Part model, mm, in its own coordinate system. A direction names the side the tool comes from. Round coordinates to 2 decimals unless told otherwise and drop trailing zeros. Order: outer loops, then holes, each group sorted by start corner. A loop starts at its lowest first (then second) coordinate and runs counter-clockwise, first axis right, second up. Notation, with made-up numbers: (-13, -31) - (-7, -31) arc R32 ccw to (-7, 1) - close; hole circle Ø7 at (15, 31). An arc over 180 degrees is marked (long way). Return JSON: item names as keys, results as strings. Group by question number.
Item 1: Probe probe 1 along X at (y, z) = (43.2, 0); probe 2 along Y at (x, z) = (-4.5, -9.5); probe 3 along Y at (x, z) = (-35.5, -7). List the from-to ranges inside material, lowest first.
Item 2: Two-plate mould, pull along Z, no slides. Class faces 4 (the face through (-76.22, 42.46, 1.15)), 5 (the face through (-19, 31, 0)), 6 (the face through (-48, 42, -18)), 7 (the face through (-3, 32, 21)): released by +Z, released by -Z, zero draft, split by the parting line, or undercut.
Item 3: Saw through at B-B on y = 35.5. List the corners of the cut face in (x, z), and give its area (3 significant figures).
Item 4: Saw through at A-A on x = -49. List the corners of the cut face in (y, z), and give its area (3 significant figures).
Item 5: Drop flat-ended pins along their axis: pin 1 (10 mm diameter, centred on y = 2.5, z = 9.5, fed in from -X); pin 2 (2 mm diameter, centred on y = 34.5, z = 20, fed in from -X); pin 3 (5 mm diameter, centred on x = -64.5, y = 41.5, fed in from -Z). Give the stop position or say it passes through.
Item 6: Saw through at D-D on y = 46. List the corners of the cut face in (x, z), and give its area (3 significant figures).
Item 7: Saw through at C-C on x = -70. List the corners of the cut face in (y, z), and give its area (3 significant figures).
Item 8: Tool access for faces 1 (the face through (-80, 42, 0)), 2 (the face through (-22.994, 30.524, -0.506)), 3 (the face through (-6, 32, 20)): list every direction of +Z, -Z, +X, -X, +Y, -Y with a clear straight run to the whole face (end or side of a thin tool).
```python
from build123d import *

# Parameters (mm, degrees)
BOSS_EXTRUDE1_DEPTH     = 62
BOSS_EXTRUDE2_START     = 3
BOSS_EXTRUDE2_DEPTH     = 3
SKETCH4_R               = 5
BOSS_EXTRUDE3_DEPTH     = 5
M6X1_0_TAPPED_HOLE1_D   = 5
CUT_EXTRUDE1_DEPTH      = 71.014284257
CUT_EXTRUDE1_DEPTH_BACK = 71.014284257
SKETCH8_W               = 3
SKETCH8_H               = 20
BOSS_EXTRUDE4_DEPTH     = 3
CUT_EXTRUDE2_REACH      = 81.919
SKETCH11_R              = 2.5
BOSS_EXTRUDE5_DEPTH     = 5
FILLET1_R               = 2


with BuildPart() as part:
    # Sketch1 → Boss-Extrude1 (new body)
    with BuildSketch(Plane(origin=(0, 0, 0), x_dir=(1, 0, 0), z_dir=(0, 1, 0))):
        with BuildLine():
            Line((0, 23), (0, 19))
            ThreePointArc((0, 19), (-19, 0), (0, -19))
            Line((0, -19), (0, -23))
            ThreePointArc((0, -23), (-23, 0), (0, 23))
        make_face()
    extrude(amount=BOSS_EXTRUDE1_DEPTH)

    # Sketch3 → Boss-Extrude2 (add)
    with BuildSketch(Plane.XZ.offset(BOSS_EXTRUDE2_START)):
        with BuildLine():
            Line((0, 23), (0, 3.75))
            ThreePointArc((0, 3.75), (-3.75, 0), (0, -3.75))
            Line((0, -3.75), (0, -23))
            ThreePointArc((0, -23), (-23, 0), (0, 23))
        make_face()
    extrude(amount=-BOSS_EXTRUDE2_DEPTH)

    # Sketch4 → Boss-Extrude3 (add)
    with BuildSketch(Plane.XZ.offset(3)):
        with Locations(Location((-10, 0, 0), (0, 0, 270))):
            Circle(SKETCH4_R)
    extrude(amount=BOSS_EXTRUDE3_DEPTH)

    # M6x1.0 Tapped Hole1 (through all)
    with Locations(Plane.XZ.offset(8)):
        with Locations((-10, 0)):
            Hole(M6X1_0_TAPPED_HOLE1_D / 2)

    # Sketch8 → Cut-Extrude1 (cut, two sides: drawn at the far end of the back side and taken through both)
    with BuildSketch(Plane.XY.offset(-CUT_EXTRUDE1_DEPTH_BACK)):
        with Locations((-4.5, 32)):
            Rectangle(SKETCH8_W, SKETCH8_H)
    extrude(amount=CUT_EXTRUDE1_DEPTH + CUT_EXTRUDE1_DEPTH_BACK, mode=Mode.SUBTRACT)

    # Sketch9 → Boss-Extrude4 (add)
    with BuildSketch(Plane(origin=(0, 62, 0), x_dir=(1, 0, 0), z_dir=(0, 1, 0))):
        with BuildLine():
            Line((0, -23), (0, 23))
            ThreePointArc((0, 23), (-23, 0), (0, -23))
        make_face()
    extrude(amount=BOSS_EXTRUDE4_DEPTH)

    # Sketch10 → Cut-Extrude2 (cut, up to next)
    with BuildSketch(Plane(origin=(0, 65, 0), x_dir=(1, 0, 0), z_dir=(0, 1, 0)), mode=Mode.PRIVATE) as cut_extrude2_sk1:
        with BuildLine():
            Line((0, -5), (-12, -5))
            ThreePointArc((-12, -5), (-17, 0), (-12, 5))
            Line((-12, 5), (0, 5))
            ThreePointArc((0, 5), (5, 0), (0, -5))
        make_face()
    cut_extrude2_tool1 = extrude(cut_extrude2_sk1.sketch, amount=-CUT_EXTRUDE2_REACH, mode=Mode.PRIVATE) & part.part
    add(cut_extrude2_tool1.solids().sort_by_distance((-6, 65, 0))[0], mode=Mode.SUBTRACT)

    # Sketch11 → Boss-Extrude5 (add)
    with BuildSketch(Plane(origin=(0, 40, 0), x_dir=(-1, 0, 0), z_dir=(0, 1, 0))):
        with BuildLine():
            Line((14.317821063, 18), (80, 18))
            Line((80, 18), (80, -18))
            Line((80, -18), (14.317821063, -18))
            ThreePointArc((14.317821063, -18), (23, 0), (14.317821063, 18))
        make_face()
        with Locations(Location((49, 0, 0), (0, 0, 90))):
            Circle(SKETCH11_R, mode=Mode.SUBTRACT)
        with Locations(Location((74, 0, 0), (0, 0, 90))):
            Circle(SKETCH11_R, mode=Mode.SUBTRACT)
    extrude(amount=BOSS_EXTRUDE5_DEPTH)

    # Fillet1
    fillet1_edges = [part.edges().sort_by_distance(p)[0] for p in [
        (-23, 40, 0),
        (-23, 45, 0),
    ]]
    fillet(fillet1_edges, radius=FILLET1_R)


solid = part.part
```
Filled in:
{
 "1": {"probe 1": "x = -80 to -76.5, -71.5 to -51.5, -46.5 to -19", "probe 2": "y = -3 to 0, 62 to 65", "probe 3": "y = 40 to 45"},
 "2": {"face 4": "undercut", "face 5": "undercut", "face 6": "released by -Z", "face 7": "zero draft"},
 "3": {"outline": "(-6, -22.2) - (-6, -18.03) arc R19 cw to (-6, 18.03) - (-6, 22.2) arc R23 ccw to start; (-3, -22.8) arc R23 ccw to (0, -23) - (0, -19) arc R19 cw to (-3, -18.76) - close; (-3, 18.76) arc R19 cw to (0, 19) - (0, 23) arc R23 ccw to (-3, 22.8) - close", "area": "239 mm^2"},
 "4": {"outline": "(40, -18) - (45, -18) - (45, -2.5) - (40, -2.5) - close; (40, 2.5) - (45, 2.5) - (45, 18) - (40, 18) - close", "area": "155 mm^2"},
 "5": {"pin 1": "stops at x = -22.56", "pin 2": "stops at x = -12.96", "pin 3": "stops at z = -18"},
 "6": {"outline": "(-14.74, -18) - (-14.32, -18) arc R23 ccw to (0, -23) - (0, -19) arc R19 cw to (0, 19) - (0, 23) arc R23 ccw to (-14.32, 18) - (-14.74, 18) arc R23.27 ccw to start", "area": "275 mm^2"},
 "7": {"outline": "(40, -18) - (45, -18) - (45, 18) - (40, 18) - close", "area": "180 mm^2"},
 "8": {"face 1": "+Z, -Z, -X, +Y, -Y", "face 2": "-X", "face 3": "+Z, -Z"}
}
